Geometry: see drawing. Coordinates: mm, zero at the bounding-box minimum. Coordinates: 2 decimals unless noted, no trailing zeros. Loops run counter-clockwise (first coordinate to the right, second up) from the corner with the lowest first, then second, coordinate; pieces in that order, holes last.
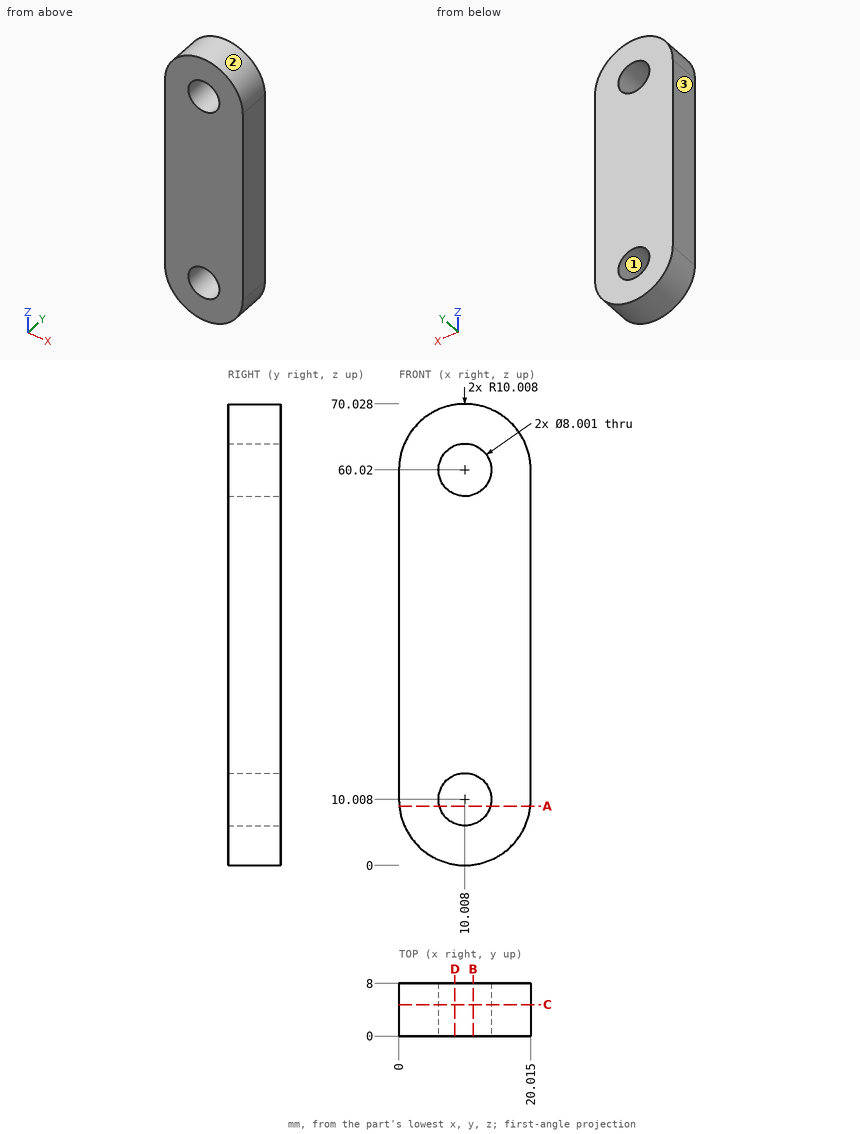
Item 1: Contact query for flat-ended pins moving along their axis: P1, Ø1, axis at y = 2, z = 7, coming from the -X side; P2, Ø1, axis at x = 17.5, y = 1, coming from the -Z side; P3, Ø1, axis at x = 7.5, y = 2, coming from the +Z side (1 decimal). Output: stop coordinate, or through.
Result:
P1: stops at x = 0.32
P2: stops at z = 2.85
P3: stops at z = 69.8
Item 2: Section query A-A (z = 9). Output: boundary loops of the cut face in (x, y) (1 decimal).
Result:
outline: (0.1, 0) - (6.1, 0) - (6.1, 8) - (0.1, 8) - close; (13.9, 0) - (20, 0) - (20, 8) - (13.9, 8) - close
Item 3: Section query C-C (y = 4.75). Output: boundary loops of the cut face in (x, z) (1 decimal).
Result:
outline: (0, 10) arc R10 ccw to (20, 10) - (20, 60) arc R10 ccw to (0, 60) - close; hole circle Ø8 at (10, 10); hole circle Ø8 at (10, 60)
Item 4: Section query B-B (x = 11.25). Count the separate pieces of the cut face and the enclosed holes in it, then the cut area to 3 significant figures.
Result:
separate pieces: 3
enclosed holes: 0
area: 437 mm2
Item 5: Mould query, pull axis Z, two halves, no side actions, for the marked faces 1, 2 and 3. Classes: +Z half, -Z half, draft (parallel to the pull), parting line (faces both ways), or undercut.
Result:
face 1: undercut
face 2: +Z half
face 3: draft
Item 6: Section query D-D (x = 8.5). Output: boundary loops of the cut face in (y, z) (1 decimal), then the cut area to 3 significant figures.
Result:
outline: (0, 0.1) - (8, 0.1) - (8, 6.3) - (0, 6.3) - close; (0, 13.7) - (8, 13.7) - (8, 56.3) - (0, 56.3) - close; (0, 63.7) - (8, 63.7) - (8, 69.9) - (0, 69.9) - close
area: 440 mm2
Item 7: Line query: L1, parallel to Z at x = 8.25, y = 3.5 (1 decimal); L2, parallel to Z at x = 12.25, y = 1 (1 decimal); L3, parallel to X at y = 5.75, z = 63.5 (1 decimal). Output: solid intervals per line, ascending.
Result:
L1: z = 0.2 to 6.4, 13.6 to 56.4, 63.6 to 69.9
L2: z = 0.3 to 6.7, 13.3 to 56.7, 63.3 to 69.8
L3: x = 0.6 to 8, 12 to 19.4
